The figure shows three views and two pictorial views of one solid part (mm, origin at its lowest corner). Answer the questions. A direction names the side the tool comes from. Round coordinates to 2 decimals unless told otherwise and drop trailing zeros. Write each loop counter-clockwise with the first axis right and the second up, starting at its lowest first coordinate (ties: lowest second). Pieces come first, ordered by that corner, then holes. Notation, with made-up numbers: (-6.5, 69) -> (8.5, 69) arc R18 ccw to (8.5, 96) -> close; hole circle Ø7 at (31.25, 41.5). An arc over 180 degrees is marked (long way). One line per item, written item: value.
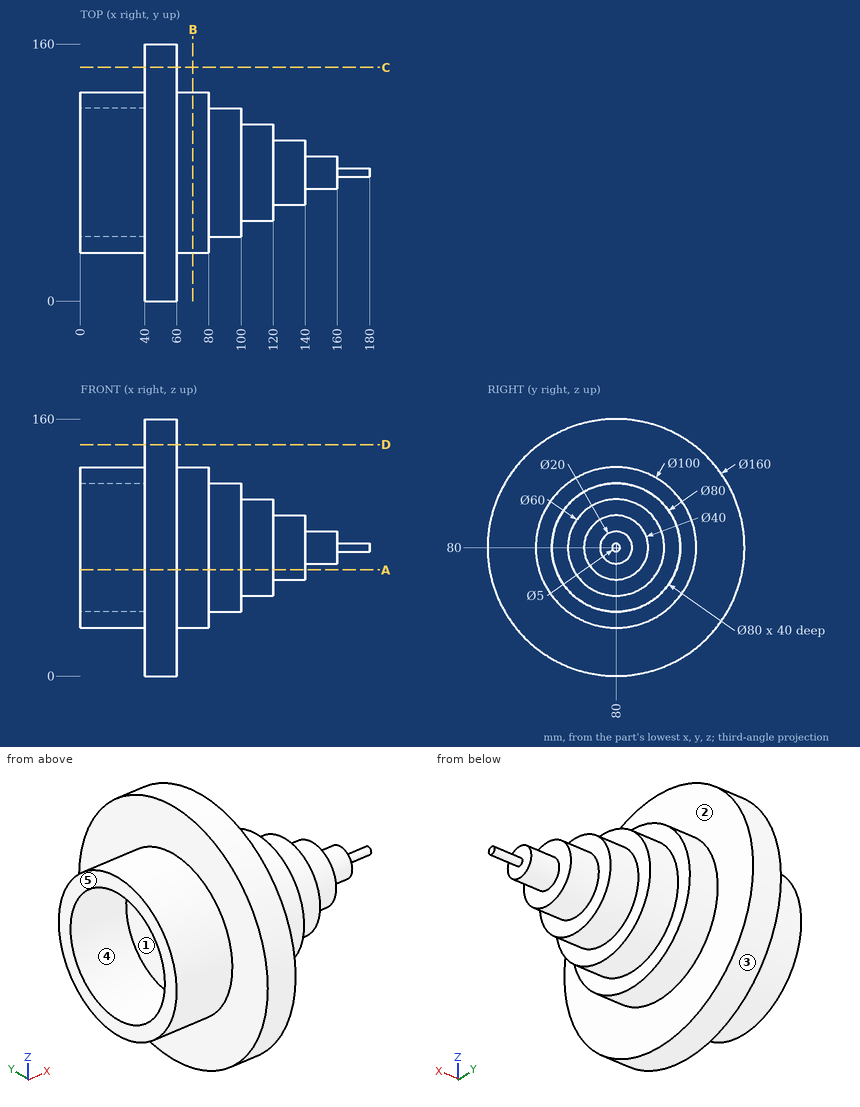
(1) A tool of negligible diameter and unlimited length cuts with its end or side. For the marked faces 1 and 2, from which of +Z, -Z, +X, -X, +Y, -Y can it reach the whole face along a straight path? Write none if from no direction.
Reported:
face 1: -X
face 2: +X
(2) Consider probe 1 along Y at (x, z) = (22, 78.5); probe 2 along X at (y, z) = (85, 21); probe 3 along Z at (x, y) = (21, 46). Determine where each line is inside the solid, lowest interval first.
Reported:
probe 1: y = 30.02 to 40.03, 119.97 to 129.98
probe 2: x = 40 to 60
probe 3: z = 43.34 to 58.93, 101.07 to 116.66
(3) Find section C-C on y = 145.5. Give the vertices of the cut face in (x, z).
Reported:
outline: (40, 34.07) -> (60, 34.07) -> (60, 125.93) -> (40, 125.93) -> close
(4) For a pull along Z with two mould halves and no side action, classify the marked faces 3, 4 and 5 as pulls with the +Z half, pulls with the -Z half, needs draft (parallel to the pull), parting line crosses it, or undercut.
Reported:
face 3: parting line crosses it
face 4: undercut
face 5: needs draft
(5) Find section A-A on z = 66. Give the vertices of the cut face in (x, y), plus the area to 3 significant figures.
Reported:
outline: (0, 32) -> (40, 32) -> (40, 1.23) -> (60, 1.23) -> (60, 32) -> (80, 32) -> (80, 42.53) -> (100, 42.53) -> (100, 53.47) -> (120, 53.47) -> (120, 65.72) -> (140, 65.72) -> (140, 94.28) -> (120, 94.28) -> (120, 106.53) -> (100, 106.53) -> (100, 117.47) -> (80, 117.47) -> (80, 128) -> (60, 128) -> (60, 158.77) -> (40, 158.77) -> (40, 128) -> (0, 128) -> (0, 117.47) -> (40, 117.47) -> (40, 42.53) -> (0, 42.53) -> close
area: 9,040 mm2
(6) Find section B-B on x = 70. Give the vertices of the cut face in (y, z), plus the area to 3 significant figures.
Reported:
outline: circle Ø100 at (80, 80)
area: 7,850 mm2
(7) Find section D-D on z = 144. Give the vertices of the cut face in (x, y).
Reported:
outline: (40, 32) -> (60, 32) -> (60, 128) -> (40, 128) -> close
(8) Flat-ended cylindrical pins translate along their axes: pin 1 Ø1.5 at (x, z) = (57, 56) entering from -Y; pin 2 Ø10 at (y, z) = (19.5, 77) entering from -X; pin 3 Ø1 at (x, z) = (89, 68.5) entering from -Y. Find the tip coordinate at first contact, or state that the pin passes through.
Reported:
pin 1: stops at y = 3.45
pin 2: stops at x = 40
pin 3: stops at y = 41.54
